Source: CAD feature listing. Evaluate the final solid. Frame: model axes, mm. Face numbers are marked on the shaded views. A direction names the side the tool comes from. Give positions to 0.01 mm unless a question says otherwise; leave off trailing zeros. Write each loop counter-clockwise with the first axis right and the second up, starting at its lowest first coordinate (ties: lowest second). Pieces come first, ordered by that corner, then holes. Notation, with made-up numbers: (20.25, -31.5) -> (45.25, -31.5) arc R32 cw to (45.25, 3.5) -> close; hole circle Ø4 at (-36.75, 64). An arc over 180 degrees is marked (long way). Use a Markdown table: item, result. Add a question column.
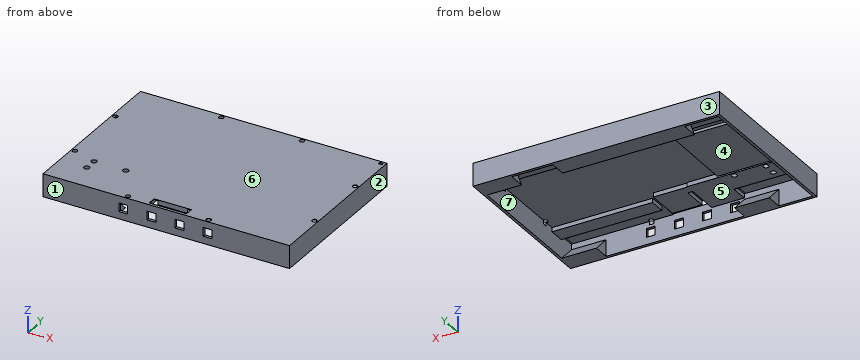
```python
from build123d import *

# Parameters (mm, degrees)
SKETCH028_W         = 178.4
SKETCH028_H         = 120.07
PAD017_DEPTH        = 1
SKETCH029_R         = 1.75
PAD018_DEPTH        = 3
SKETCH026_W         = 32
SKETCH026_H         = 18
PAD015_DEPTH        = 1
SKETCH027_R         = 2
PAD016_DEPTH        = 10
SKETCH002_W         = 178.4
SKETCH002_H         = 120.07
SKETCH002_W_2       = 26.9298
SKETCH002_H_2       = 6
PAD002_DEPTH        = 0.5
SKETCH003_W         = 178.4
SKETCH003_H         = 120.07
SKETCH003_W_2       = 174.4
SKETCH003_H_2       = 116.07
PAD003_DEPTH        = 16
PAD004_DEPTH        = 25
LINEARPATTERN_COUNT = 2
LINEARPATTERN_PITCH = 125
SKETCH012_R         = 0.8
POCKET002_DEPTH     = 2.5
SKETCH013_W         = 2.5
SKETCH013_H         = 1.8
POCKET003_DEPTH     = 2
SKETCH017_W         = 6.3
SKETCH017_H         = 6.3
POCKET004_DEPTH     = 5
PAD010_DEPTH        = 2
SKETCH019_W         = 15.51
SKETCH019_H         = 1
POCKET005_DEPTH     = 0.5
SKETCH020_W         = 70.44
SKETCH020_H         = 12
PAD011_DEPTH        = 16
PAD012_DEPTH        = 12
PAD013_DEPTH        = 12
SKETCH025_W         = 21.22
SKETCH025_H         = 23.77
SKETCH025_W_2       = 3.5749
SKETCH025_H_2       = 6.45
SKETCH025_W_3       = 72.78
SKETCH025_H_3       = 11.45
SKETCH025_W_4       = 174.4
SKETCH025_H_4       = 11.68
SKETCH025_W_5       = 70.43
SKETCH025_H_5       = 0.7
PAD014_DEPTH        = 3


with BuildPart() as holes_bezel:
    # Sketch028 (on Face1 of Binder013) → Pad017 (new body)
    with BuildSketch(Plane(origin=(0, 0, -0.41), x_dir=(1, 0, 0), z_dir=(0, 0, -1))):
        with Locations((0, 0.305)):
            Rectangle(SKETCH028_W, SKETCH028_H)
    extrude(amount=-PAD017_DEPTH)

    # Sketch029 (on Face5 of Pad017) → Pad018 (join)
    with BuildSketch(Plane(origin=(0, 0, -0.41), x_dir=(1, 0, 0), z_dir=(0, 0, -1))):
        with Locations((29.2, 57.84)):
            Circle(SKETCH029_R)
        with Locations((-29.2, 57.84)):
            Circle(SKETCH029_R)
        with Locations((86.7, 25.34)):
            Circle(SKETCH029_R)
        with Locations((86.7, -24.73)):
            Circle(SKETCH029_R)
        with Locations((29.2, -57.23)):
            Circle(SKETCH029_R)
        with Locations((-29.2, -57.23)):
            Circle(SKETCH029_R)
        with Locations((-86.7, -24.73)):
            Circle(SKETCH029_R)
        with Locations((-86.7, 25.34)):
            Circle(SKETCH029_R)
    extrude(amount=PAD018_DEPTH)


with BuildPart() as holes:
    # Sketch026 (on Face9 of Binder011) → Pad015 (new body)
    with BuildSketch(Plane(origin=(0, 0, -6.91), x_dir=(1, 0, 0), z_dir=(0, 0, -1))):
        with Locations((-58.15, 35.24)):
            Rectangle(SKETCH026_W, SKETCH026_H)
    extrude(amount=PAD015_DEPTH)

    # Sketch027 (on Face5 of Pad015) → Pad016 (join)
    with BuildSketch(Plane.XY.offset(-6.91)):
        with Locations((-69.65, -30.74)):
            Circle(SKETCH027_R)
        with Locations((-46.65, -30.74)):
            Circle(SKETCH027_R)
        with Locations((-69.65, -39.74)):
            Circle(SKETCH027_R)
    extrude(amount=PAD016_DEPTH)


with BuildPart() as cut_case:
    # Sketch002 (on Face1 of Binder001) → Pad002 (new body)
    with BuildSketch(Plane(origin=(0, 0, -0.41), x_dir=(1, 0, 0), z_dir=(0, 0, -1))):
        with Locations((0, 0.305)):
            Rectangle(SKETCH002_W, SKETCH002_H)
        with Locations((0, 55.34)):
            Rectangle(SKETCH002_W_2, SKETCH002_H_2, mode=Mode.SUBTRACT)
    extrude(amount=PAD002_DEPTH)

    # Sketch003 (on Face10 of Pad002) → Pad003 (join)
    with BuildSketch(Plane(origin=(0, 0, -0.91), x_dir=(1, 0, 0), z_dir=(0, 0, -1))):
        with Locations((0, 0.305)):
            Rectangle(SKETCH003_W, SKETCH003_H)
        with Locations((0, 0.305)):
            Rectangle(SKETCH003_W_2, SKETCH003_H_2, mode=Mode.SUBTRACT)
    extrude(amount=PAD003_DEPTH)

    # Sketch004 (on Face9 of Pad003) → Pad004 (join)
    with BuildSketch(Plane(origin=(87.2, 0, 0), x_dir=(0, -1, 0), z_dir=(-1, 0, 0))):
        Polygon((-57.73, -16.91), (-57.73, -4.91), (-45.73, -16.91), align=None)
        Polygon((58.34, -16.91), (58.34, -4.91), (46.34, -16.91), align=None)
    pad004 = extrude(amount=PAD004_DEPTH)

    # LinearPattern: Pad004 ×2
    with Locations(*[(-i * LINEARPATTERN_PITCH, 0, 0) for i in range(1, LINEARPATTERN_COUNT)]):
        add(pad004)

    # Sketch012 (on Face1 of LinearPattern) → Pocket002 (cut)
    with BuildSketch(Plane.XY.offset(-0.41)):
        with Locations((-86.7, 24.73)):
            Circle(SKETCH012_R)
        with Locations((-86.7, -25.34)):
            Circle(SKETCH012_R)
        with Locations((-29.2, -57.84)):
            Circle(SKETCH012_R)
        with Locations((29.2, -57.84)):
            Circle(SKETCH012_R)
        with Locations((86.7, -25.34)):
            Circle(SKETCH012_R)
        with Locations((86.7, 24.73)):
            Circle(SKETCH012_R)
        with Locations((29.2, 57.23)):
            Circle(SKETCH012_R)
        with Locations((-29.2, 57.23)):
            Circle(SKETCH012_R)
    extrude(amount=-POCKET002_DEPTH, mode=Mode.SUBTRACT)

    # Sketch013 (on Face1 of Pocket002) → Pocket003 (cut)
    with BuildSketch(Plane.XY.offset(-0.41)):
        with Locations((86.14, 57.44)):
            Rectangle(SKETCH013_W, SKETCH013_H)
    extrude(amount=-POCKET003_DEPTH, mode=Mode.SUBTRACT)

    # Sketch017 (on Face3 of Pocket003) → Pocket004 (cut)
    with BuildSketch(Plane.XZ.offset(60.34)):
        with Locations((-31.05, -8.56)):
            Rectangle(SKETCH017_W, SKETCH017_H)
        with Locations((-10.75, -8.56)):
            Rectangle(SKETCH017_W, SKETCH017_H)
        with Locations((9.55, -8.56)):
            Rectangle(SKETCH017_W, SKETCH017_H)
        with Locations((29.85, -8.56)):
            Rectangle(SKETCH017_W, SKETCH017_H)
    extrude(amount=-POCKET004_DEPTH, mode=Mode.SUBTRACT)

    # Sketch018 (on Face39 of Pocket004) → Pad010 (join)
    with BuildSketch(Plane(origin=(0, 0, -0.91), x_dir=(1, 0, 0), z_dir=(0, 0, -1))):
        Polygon((-87.2, 29.22), (-87.2, -25.72), (-36.679044, -25.72), (-36.19, 29.22), align=None)
    extrude(amount=PAD010_DEPTH)

    # Sketch019 (on Face42 of Pad010) → Pocket005 (cut)
    with BuildSketch(Plane(origin=(87.2, 0, 0), x_dir=(0, -1, 0), z_dir=(-1, 0, 0))):
        with Locations((-50.085, -1.41)):
            Rectangle(SKETCH019_W, SKETCH019_H)
    extrude(amount=-POCKET005_DEPTH, mode=Mode.SUBTRACT)

    # Sketch020 (on Face74 of Pocket005) → Pad011 (join)
    with BuildSketch(Plane(origin=(0, 0, -0.91), x_dir=(1, 0, 0), z_dir=(0, 0, -1))):
        with Locations((-2.58, -51.73)):
            Rectangle(SKETCH020_W, SKETCH020_H)
    extrude(amount=PAD011_DEPTH)

    # Sketch022 (on Face69 of Pad011) → Pad012 (join)
    with BuildSketch(Plane.XZ.offset(-57.73)):
        Polygon((-38.8, -0.91), (-37.8, -1.11), (-37.8, -0.91), align=None)
        Polygon((84.89, -1.06), (83.89, -0.91), (84.89, -0.91), align=None)
    extrude(amount=PAD012_DEPTH)

    # Sketch023 (on Face10 of Pad012) → Pad013 (join)
    with BuildSketch(Plane(origin=(0, -58.34, 0), x_dir=(-1, 0, 0), z_dir=(0, 1, 0))):
        Polygon((37.8, -0.91), (38.8, -0.91), (37.8, -1.11), align=None)
        Polygon((-87.2, -0.91), (-86.2, -0.91), (-87.2, -1.11), align=None)
    extrude(amount=PAD013_DEPTH)

    # Sketch025 (on Face39 of Pad013) → Pad014 (join)
    with BuildSketch(Plane(origin=(0, 0, -0.91), x_dir=(1, 0, 0), z_dir=(0, 0, -1))):
        with Locations((0, 40.455)):
            Rectangle(SKETCH025_W, SKETCH025_H)
        Polygon((-14.1849, 27.96), (-87.2, 27.96), (-87.2, 45.64), (-37.8, 45.64), (-37.8, 58.34), (-14.1849, 58.34), align=None)
        with Locations((-12.39745, 31.795)):
            Rectangle(SKETCH025_W_2, SKETCH025_H_2)
        with Locations((50.81, 39.915)):
            Rectangle(SKETCH025_W_3, SKETCH025_H_3)
        with Locations((0, -39.19)):
            Rectangle(SKETCH025_W_4, SKETCH025_H_4)
        with Locations((-2.575, -45.38)):
            Rectangle(SKETCH025_W_5, SKETCH025_H_5)
    extrude(amount=PAD014_DEPTH)

    # Cut: cut holes
    add(holes.part, mode=Mode.SUBTRACT)

    # Cut001: cut holes bezel
    add(holes_bezel.part, mode=Mode.SUBTRACT)


solid = cut_case.part
```
(1) Cut plane B-B on x = -46.65. Return the cut outline in (y, z), then the cut area to 3 significant figures.
(2) Cut plane A-A on y = -39.74. Return the cut outline in (x, z), then the cut area to 3 significant figures.
(3) Access query for the marked faces 5, 6 and 7. Directions: +Z, -Z, +X, -X, +Y, -Y. A direction counts if a zero-diameter tool reaches every point of the face in a straight line with its end or side. Return the directions, or none.
(4) Material intervals for L1, parallel to Y at x = -86.7, z = -2.5; L2, parallel to Y at x = -46.65, z = -2.65; L3, parallel to X at y = -30.74, z = -2.55, sorted ascending.
(5) Mould query, pull axis Y, two halves, no side actions, for the marked faces 1, 2, 3 and 4. Classes: +Y half, -Y half, draft (parallel to the pull), parting line (faces both ways), or undercut.
(6) Cut plane C-C on z = -15. Return the cut outline in (x, y).
(7) First-contact query: pin 1 Ø0.9 at (x, y) = (86.5, 57.5) entering from +Z; pin 2 Ø1 at (x, y) = (28.5, 56.5) entering from +Z; pin 3 Ø10 at (x, y) = (71, -36) entering from -Z. Flat tips, straight axial feed; report the tip coordinate or a pass-through.
(8) Cut plane D-D on x = 43. Return the cut outline in (y, z), then the cut area to 3 significant figures.
Output:
| question | item | result |
|---|---|---|
| 1 | outline | (-60.34, -16.91) -> (-46.34, -16.91) -> (-58.34, -4.91) -> (-58.34, -0.91) -> (-45.64, -0.91) -> (-45.64, -3.91) -> (-32.74, -3.91) -> (-32.74, -0.41) -> (-60.34, -0.41) -> close; (-28.74, -3.91) -> (-27.96, -3.91) -> (-27.96, -2.91) -> (25.72, -2.91) -> (25.72, -0.91) -> (33.35, -0.91) -> (33.35, -3.91) -> (45.03, -3.91) -> (45.03, -0.91) -> (57.73, -0.91) -> (57.73, -4.91) -> (45.73, -16.91) -> (59.73, -16.91) -> (59.73, -0.41) -> (-28.74, -0.41) -> close |
| 1 | area | 449 mm^2 |
| 2 | outline | (-89.2, -16.91) -> (-87.2, -16.91) -> (-87.2, -3.91) -> (-71.65, -3.91) -> (-71.65, -0.41) -> (-89.2, -0.41) -> close; (-67.65, -3.91) -> (-14.18, -3.91) -> (-14.18, -0.91) -> (-10.61, -0.91) -> (-10.61, -3.91) -> (10.61, -3.91) -> (10.61, -0.91) -> (14.42, -0.91) -> (14.42, -3.91) -> (87.2, -3.91) -> (87.2, -16.91) -> (89.2, -16.91) -> (89.2, -0.41) -> (-67.65, -0.41) -> close |
| 2 | area | 640 mm^2 |
| 3 | face 5 | -Z |
| 3 | face 6 | +Z, +X, -X, +Y, -Y |
| 3 | face 7 | none |
| 4 | L1 | -60.34 to -58.34, -45.64 to -27.09, -23.59 to 22.98, 33.35 to 45.03, 57.73 to 59.73 |
| 4 | L2 | -60.34 to -58.34, -45.64 to -32.74, -28.74 to 25.72, 33.35 to 45.03, 57.73 to 59.73 |
| 4 | L3 | -89.2 to -71.65, -67.65 to -48.65, -44.65 to 10.61, 87.2 to 89.2 |
| 5 | face 1 | -Y half |
| 5 | face 2 | draft |
| 5 | face 3 | +Y half |
| 5 | face 4 | undercut |
| 6 | outline | (-89.2, -60.34) -> (89.2, -60.34) -> (89.2, 59.73) -> (-89.2, 59.73) -> close; hole (-87.2, -58.34) -> (-62.8, -58.34) -> (-62.8, -48.25) -> (-37.8, -48.25) -> (-37.8, -58.34) -> (62.2, -58.34) -> (62.2, -48.25) -> (87.2, -48.25) -> (87.2, 47.64) -> (62.2, 47.64) -> (62.2, 57.73) -> (32.64, 57.73) -> (32.64, 45.73) -> (-37.8, 45.73) -> (-37.8, 47.64) -> (-62.8, 47.64) -> (-62.8, 57.73) -> (-87.2, 57.73) -> close |
| 7 | pin 1 | z = -2.41 |
| 7 | pin 2 | z = -3.41 |
| 7 | pin 3 | z = -3.91 |
| 8 | outline | (-60.34, -16.91) -> (-58.34, -16.91) -> (-58.34, -0.91) -> (-45.64, -0.91) -> (-45.64, -3.91) -> (-34.19, -3.91) -> (-34.19, -0.91) -> (33.35, -0.91) -> (33.35, -3.91) -> (45.03, -3.91) -> (45.03, -0.91) -> (57.73, -0.91) -> (57.73, -16.91) -> (59.73, -16.91) -> (59.73, -0.41) -> (-60.34, -0.41) -> close |
| 8 | area | 193 mm^2 |
